Check sheet for the modelled part. Datum: model origin and axes. Units: mm. A direction names the side the tool comes from. Round coordinates to 2 decimals unless told otherwise and drop trailing zeros. Loops run counter-clockwise (first coordinate to the right, second up) from the corner with the lowest first, then second, coordinate; pieces in that order, holes last. Notation, with made-up numbers: (59.25, 4.25) -> (104.25, 4.25) arc R13 cw to (104.25, 27.25) -> close; hole circle Ø6 at (-30, 71). An arc over 180 degrees is marked (long way). Return JSON: item names as keys, results as strings.
from build123d import *

# Parameters (mm, degrees)
SKETCH_1_W          = 10
SKETCH_1_H          = 10
SKETCH_1_W_2        = 8
SKETCH_1_H_2        = 8
EXTRUDE_1_DEPTH     = 175
SKETCH_2_R          = 1.5
CUT_EXTRUDE_1_DEPTH = 11
SKETCH_3_R          = 1.5
CUT_EXTRUDE_2_DEPTH = 10


with BuildPart() as part:
    # 草图1 → 拉伸-薄壁1 (new body)
    with BuildSketch(Plane.XY):
        Rectangle(SKETCH_1_W, SKETCH_1_H)
        Rectangle(SKETCH_1_W_2, SKETCH_1_H_2, mode=Mode.SUBTRACT)
    extrude(amount=EXTRUDE_1_DEPTH)

    # 草图2 → 切除-拉伸1 (cut, through all)
    with BuildSketch(Plane(origin=(5, 0, 0), x_dir=(0, 0, -1), z_dir=(1, 0, 0))):
        with Locations((-80, 0)):
            Circle(SKETCH_2_R)
        with Locations((-115, 0)):
            Circle(SKETCH_2_R)
        with Locations((-145, 0)):
            Circle(SKETCH_2_R)
    extrude(amount=-CUT_EXTRUDE_1_DEPTH, mode=Mode.SUBTRACT)

    # 草图3 → 切除-拉伸2 (cut)
    with BuildSketch(Plane(origin=(0, 5, 0), x_dir=(1, 0, 0), z_dir=(0, 1, 0))):
        with Locations((0, -5)):
            Circle(SKETCH_3_R)
        with Locations((0, -45)):
            Circle(SKETCH_3_R)
        Polygon((5, -165), (5, -175), (-5, -175), align=None)
    extrude(amount=-CUT_EXTRUDE_2_DEPTH, mode=Mode.SUBTRACT)


solid = part.part
Q1. Go/stop test with flat-tipped pins: pin 1 (2.5 mm diameter, centred on y = 0, z = 145, fed in from +X); pin 2 (3.5 mm diameter, centred on x = 0, z = 5, fed in from -Y); pin 3 (2 mm diameter, centred on x = -3.5, y = 3, fed in from +Z). Record where each tip stops, or that it passes through.
Results list:
{"pin 1": "through", "pin 2": "y = -5", "pin 3": "z = 174.5"}
Q2. Draft check along X on faces 3 (the flat face through (0, -5, 86)), 4 (the flat face through (5, 1.04, 81.34)), 5 (the flat face through (0, 4, 86)), 6 (the flat face through (0, -4, 86)). Enter one of: released by +X, released by -X, zero draft, split by the parting line, or undercut.
Results list:
{"face 3": "zero draft", "face 4": "released by +X", "face 5": "undercut", "face 6": "undercut"}
Q3. Material ranges on line 1 (X direction, y = 3.75, z = 36); line 2 (X direction, y = 4.75, z = 45), recorded low to high.
Results list:
{"line 1": "-5 to -4, 4 to 5", "line 2": "-5 to -1.5, 1.5 to 5"}
Q4. Tool access check on faces 1 (the flat face through (-5, 0, 86)), 2 (the flat face through (-4, 0, 86)). Record the directions out of +Z, -Z, +X, -X, +Y, -Y that give a thin tool (end or side, any length) a straight path to the whole face; none if there is none.
Results list:
{"face 1": "+Z, -Z, -X, +Y, -Y", "face 2": "+Z, -Z"}
Q5. Section check B-B (x = 0). Record the boundary of the cut face in (y, z), then the cut area to 3 significant figures.
Results list:
{"outline": "(-5, 0) -> (-4, 0) -> (-4, 3.5) -> (-5, 3.5) -> close; (-5, 6.5) -> (-4, 6.5) -> (-4, 43.5) -> (-5, 43.5) -> close; (-5, 46.5) -> (-4, 46.5) -> (-4, 170) -> (-5, 170) -> close; (4, 0) -> (5, 0) -> (5, 3.5) -> (4, 3.5) -> close; (4, 6.5) -> (5, 6.5) -> (5, 43.5) -> (4, 43.5) -> close; (4, 46.5) -> (5, 46.5) -> (5, 170) -> (4, 170) -> close", "area": "328 mm^2"}
Q6. Section check A-A (z = 115). Record the boundary of the cut face in (x, y).
Results list:
{"outline": "(-5, -5) -> (5, -5) -> (5, -1.5) -> (4, -1.5) -> (4, -4) -> (-4, -4) -> (-4, -1.5) -> (-5, -1.5) -> close; (-5, 1.5) -> (-4, 1.5) -> (-4, 4) -> (4, 4) -> (4, 1.5) -> (5, 1.5) -> (5, 5) -> (-5, 5) -> close"}
